Autodesk Inventor part; units mm, degrees
ref_plane "YZ Plane" through (0, 0, 0) normal (1, 0, 0) x (0, 1, 0)
ref_plane "XZ Plane" through (0, 0, 0) normal (0, 1, 0) x (-1, 0, 0)
ref_plane "XY Plane" through (0, 0, 0) normal (0, 0, 1) x (1, 0, 0)
sketch "Sketch1" plane through (0, 0, 0) normal (0, 1, 0) x (-1, 0, 0)
  circle A0 centre (0, 0) radius 5
  line L0 (5, 0) -> (9.8774, -1.3309) construction
  arc A1 (8.2733, -0.1123) -> (3.8334, 0.4702) centre (4.1778, -14.1163) ccw
  line L1 (9.8774, -1.3309) -> (5, 0) construction
  arc A2 (3.8334, -1.3043) -> (8.2733, -0.7218) centre (4.1778, 13.2822) ccw
  line L2 (3.8879, -2.2603) -> (3.8879, -0.5721)
  line L3 (3.8879, -0.262) -> (3.8879, 1.4262)
  line L4 (0.1623, -0.03) -> (0.1623, 0.0204)
  circle A3 centre (0, 0) radius 2.75
  line L5 (8.2733, -0.7218) -> (8.2733, -0.1123)
  arc A4 (3.972, 0.7871) -> (7.5258, 3.5116) centre (-3.023, 13.5916) ccw
  line L6 (7.5258, 3.5116) -> (7.2211, 4.0394)
  arc A5 (7.2211, 4.0394) -> (3.0847, 2.3239) centre (10.6762, -10.1362) ccw
  arc A6 (3.0463, 2.6677) -> (4.7618, 6.804) centre (-9.4138, 10.2592) ccw
  line L7 (4.7618, 6.804) -> (4.2339, 7.1088)
  arc A7 (4.2339, 7.1088) -> (1.5095, 3.5549) centre (14.314, -3.4401) ccw
  arc A8 (1.3043, 3.8334) -> (0.7218, 8.2733) centre (-13.2822, 4.1778) ccw
  line L8 (0.7218, 8.2733) -> (0.1123, 8.2733)
  arc A9 (0.1123, 8.2733) -> (-0.4702, 3.8334) centre (14.1163, 4.1778) ccw
  arc A10 (-0.7871, 3.972) -> (-3.5116, 7.5258) centre (-13.5916, -3.023) ccw
  line L9 (-3.5116, 7.5258) -> (-4.0394, 7.2211)
  arc A11 (-4.0394, 7.2211) -> (-2.3239, 3.0847) centre (10.1362, 10.6762) ccw
  arc A12 (-2.6677, 3.0463) -> (-6.804, 4.7618) centre (-10.2592, -9.4138) ccw
  line L10 (-6.804, 4.7618) -> (-7.1088, 4.2339)
  arc A13 (-7.1088, 4.2339) -> (-3.5549, 1.5095) centre (3.4401, 14.314) ccw
  arc A14 (-3.8334, 1.3043) -> (-8.2733, 0.7218) centre (-4.1778, -13.2822) ccw
  line L11 (-8.2733, 0.7218) -> (-8.2733, 0.1123)
  arc A15 (-8.2733, 0.1123) -> (-3.8334, -0.4702) centre (-4.1778, 14.1163) ccw
  arc A16 (-3.972, -0.7871) -> (-7.5258, -3.5116) centre (3.023, -13.5916) ccw
  line L12 (-7.5258, -3.5116) -> (-7.2211, -4.0394)
  arc A17 (-7.2211, -4.0394) -> (-3.0847, -2.3239) centre (-10.6762, 10.1362) ccw
  arc A18 (-3.0463, -2.6677) -> (-4.7618, -6.804) centre (9.4138, -10.2592) ccw
  line L13 (-4.7618, -6.804) -> (-4.2339, -7.1088)
  arc A19 (-4.2339, -7.1088) -> (-1.5095, -3.5549) centre (-14.314, 3.4401) ccw
  arc A20 (-1.3043, -3.8334) -> (-0.7218, -8.2733) centre (13.2822, -4.1778) ccw
  line L14 (-0.7218, -8.2733) -> (-0.1123, -8.2733)
  arc A21 (-0.1123, -8.2733) -> (0.4702, -3.8334) centre (-14.1163, -4.1778) ccw
  arc A22 (0.7871, -3.972) -> (3.5116, -7.5258) centre (13.5916, 3.023) ccw
  line L15 (3.5116, -7.5258) -> (4.0394, -7.2211)
  arc A23 (4.0394, -7.2211) -> (2.3239, -3.0847) centre (-10.1362, -10.6762) ccw
  arc A24 (2.6677, -3.0463) -> (6.804, -4.7618) centre (10.2592, 9.4138) ccw
  line L16 (6.804, -4.7618) -> (7.1088, -4.2339)
  arc A25 (7.1088, -4.2339) -> (3.5549, -1.5095) centre (-3.4401, -14.314) ccw
  point P0 (4.8297, -1.2938)
  point P1 (4.9795, 0.4523)
  point P2 (4.0863, 2.8814)
  point P3 (4.8296, 1.2944)
  point P4 (2.0981, 4.5385)
  point P5 (3.5353, 3.5357)
  point P6 (-0.4523, 4.9795)
  point P7 (1.2938, 4.8297)
  point P8 (-2.8814, 4.0863)
  point P9 (-1.2944, 4.8296)
  point P10 (-4.5385, 2.0981)
  point P11 (-3.5357, 3.5353)
  point P12 (-4.9795, -0.4523)
  point P13 (-4.8297, 1.2938)
  point P14 (-4.0863, -2.8814)
  point P15 (-4.8296, -1.2944)
  point P16 (-2.0981, -4.5385)
  point P17 (-3.5353, -3.5357)
  point P18 (0.4523, -4.9795)
  point P19 (-1.2938, -4.8297)
  point P20 (2.8814, -4.0863)
  point P21 (1.2944, -4.8296)
  point P22 (4.5385, -2.0981)
  point P23 (3.5357, -3.5353)
  dimension "d0" = 10
  dimension "d5" = 5.5
  dimension "d14" = 360
extrude "Extrusion1" add sketch "Sketch1" along normal blind 5
sketch "Sketch2" plane through (0, 5, 0) normal (0, 1, 0) x (1, 0, 0)
  line L0 (-2.3094, 4) -> (2.3094, 4)
  line L1 (2.3094, 4) -> (4.6188, 0)
  line L2 (4.6188, 0) -> (2.3094, -4)
  line L3 (2.3094, -4) -> (-2.3094, -4)
  line L4 (-2.3094, -4) -> (-4.6188, 0)
  line L5 (-4.6188, 0) -> (-2.3094, 4)
  line L6 (0, 0) -> (-6.3613, 0)
  dimension "d8" = 8
extrude "Extrusion2" cut sketch "Sketch2" against normal blind 1
ref_plane "Work Plane1" through (0, 2.5, 0) normal (0, 1, 0) x (1, 0, 0)
mirror "Mirror1" about plane through (0, 2.5, 0) normal (0, 1, 0) of "Extrusion2"
properties part number "JointFixeSmallr"
For this review, take the finished solid that the model builds, in its own axes (mm). A direction names the side the tool comes from. Round coordinates to 2 decimals unless told otherwise and drop trailing zeros. Loops run counter-clockwise (first coordinate to the right, second up) from the corner with the lowest first, then second, coordinate; pieces in that order, holes last. Notation, with made-up numbers: (-9.75, 74) - (6.25, 74) arc R25 ccw to (6.25, 110) - close; hole circle Ø7 at (72.5, 56). An arc over 180 degrees is marked (long way). Put each result on its own line as item: value. Start each with the question number.
1. Consider section A-A on x = -1. State the section outline as (y, z) points.
2. Insertion check: P1, Ø2.5, axis at x = 1.5, z = -1.5, coming from the -Y side; P2, Ø2, axis at x = 3.5, y = 1, coming from the -Z side. Each pin has a flat end and moves straight along its axis. Give the tip position at first contact, or say it passes through.
3. Mouldability with a two-part tool opening along X and no side actions: class faces 1 (the cylindrical face through (-6.62, 2.46, 0.27)), 2 (the cylindrical face through (-2.338, 2.465, -6.263)), 3 (the cylindrical face through (4.92, 2.46, -0.88)) as +X half, -X half, draft (parallel to the pull), parting line (faces both ways), or undercut.
4. For faces 4 (the cylindrical face through (2.338, 2.465, 6.263)), 5 (the flat face through (3.48, 4.51, 1.97)), 6 (the cylindrical face through (5.598, 2.465, -3.542)), 7 (the cylindrical face through (6.62, 2.46, -0.27)), list the 3-axis set-ups (+Z, -Z, +X, -X, +Y, -Y) from which the entire face can be reached by the end or side of a thin tool; tool diameter is ignored.
5. Consider section B-B on x = 6.5. State the section outline as (y, z) points, plus the area to 3 significant figures.
6. For probe 1 along X at (y, z) = (4.4, 3.25); probe 2 along Z at (x, y) = (3, 0.95); probe 3 along Z at (x, y) = (7, 3.6), list the stretches that pass through material, from the lowest coordinate up. Write a range as [from, to].
Result sheet:
1. outline: (0, -4.9) - (5, -4.9) - (5, -4) - (4, -4) - (4, -2.56) - (1, -2.56) - (1, -4) - (0, -4) - close; (0, 4) - (1, 4) - (1, 2.56) - (4, 2.56) - (4, 4) - (5, 4) - (5, 7.16) - (0, 7.16) - close
2. P1: y = 1
2. P2: z = -7.11
3. face 1: -X half
3. face 2: undercut
3. face 3: +X half
4. face 4: +Z, +Y, -Y
4. face 5: +Y
4. face 6: +Y, -Y
4. face 7: +X, +Y, -Y
5. outline: (0, -3.84) - (5, -3.84) - (5, -2.54) - (0, -2.54) - close; (0, -0.29) - (5, -0.29) - (5, 1.12) - (0, 1.12) - close; (0, 3.63) - (5, 3.63) - (5, 4.68) - (0, 4.68) - close
5. area: 18.8 mm^2
6. probe 1: [-7.27, -4.87], [-3.8, -2.74], [2.74, 6.07]
6. probe 2: [-5.77, -2.8], [2.8, 4], [4.33, 7.01]
6. probe 3: [-3.98, -2.99], [-0.2, 1.03], [4.12, 4.42]
